Read the model definition and answer for the solid it produces. Units are mm, in the model's axes. A direction names the side the tool comes from. Coordinates: 2 decimals unless noted, no trailing zeros. Loops run counter-clockwise (first coordinate to the right, second up) from the corner with the lowest first, then second, coordinate; pieces in that order, holes last. Notation, with made-up numbers: (66.5, 9.25) -> (105.5, 9.25) arc R18 cw to (105.5, 17.25) -> close; hole circle Ø1 at (46, 35). An arc over 180 degrees is marked (long way). Answer as a JSON object with one key per item and string values. Group by question number.
Q1. The part is cut by section A-A on z = 0. Write down the section's boundary in (x, y).
Q2. The part is cut by section D-D on y = 25. Write down the section's boundary in (x, z), and give its area (3 significant figures).
Q3. Each of these flat-tipped pins is pushed along its axis until it touches: P1, Ø1, axis at x = 7.5, y = -24.5, coming from the +Z side; P2, Ø14, axis at y = -2.5, z = -1, coming from the +X side; P3, Ø8, axis at x = 9, y = -20.5, coming from the +Z side; P4, Ø3, axis at x = 5, y = 0.5, coming from the +Z side. Where does it stop, or does it pass through?
Q4. For faces 1 (the cylindrical face through (5.07, -29.25, 23.53)), 2 (the cylindrical face through (12.958, 27.334, -6.07)), determine the directions among +Z, -Z, +X, -X, +Y, -Y from which every point of the face is accessible in a straight line to the end or side of a thin tool.
Q5. The part is cut by section B-B on y = 0. Write down the section's boundary in (x, z).
Q6. The part is cut by section C-C on z = 35. Write down the section's boundary in (x, y).
Q7. Determine the mould class of faces 3 (the cylindrical face through (5.07, -26.429, -23.033)), 4 (the flat face through (0, 9, -1)), 5 (the cylindrical face through (4.93, 25.861, -33.727)) for opening direction Y: released by +Y, released by -Y, zero draft, split by the parting line, or undercut.
Q8. Straight lines are drawn through the part: line 1 along Y through (x, z) = (13.75, -16.5); line 2 along Y through (x, z) = (13.5, 0); line 3 along Z through (x, y) = (6.25, -31). For each, find the intervals that lie inside material, in ascending order. Write a range as [from, to].
from build123d import *

# Parameters (mm, degrees)
HOLE_WIZARD_6_0_6_1_D = 6.2


with BuildPart() as part:
    # Эскиз1 → Повернуть1 (revolve)
    with BuildSketch(Plane.XY, mode=Mode.PRIVATE) as revolve_1_sk:
        Polygon((0, -2), (8, -2), (8, -23), (16, -23), (16, -28), (10, -28), (10, -42.5), (0, -42.5), align=None)
    revolve(revolve_1_sk.sketch.rotate(Axis((-696.045801993, 0, 0), (1, 0, 0)), 270), axis=Axis((-696.045801993, 0, 0), (1, 0, 0)))

    # Диаметр отверстия Ø6.0 (6)1 (through all)
    with Locations(Plane(origin=(0, 10.815594803, -33.28697807), x_dir=(0, 0, -1), z_dir=(-1, 0, 0))):
        with Locations((0, 0), (-66.57395614, 0), (-33.28697807, -24.184405197), (-12.71449424, 39.131189606), (-53.8594619, 39.131189606)):
            Hole(HOLE_WIZARD_6_0_6_1_D / 2)


solid = part.part
Final values:
{
 "1": {"outline": "(0, -42.5) -> (10, -42.5) -> (10, -28) -> (16, -28) -> (16, -23) -> (8, -23) -> (8, -2) -> (0, -2) -> close; (0, 2) -> (8, 2) -> (8, 23) -> (16, 23) -> (16, 28) -> (10, 28) -> (10, 31.9) -> (0, 31.9) -> close; (0, 38.1) -> (10, 38.1) -> (10, 42.5) -> (0, 42.5) -> close"},
 "2": {"outline": "(0, -34.37) -> (10, -34.37) -> (10, -12.61) -> (16, -12.61) -> (16, 12.61) -> (10, 12.61) -> (10, 34.37) -> (0, 34.37) -> close", "area": "839 mm2"},
 "3": {"P1": "stops at z = 35.07", "P2": "stops at x = 8", "P3": "stops at z = 39.17", "P4": "stops at z = 42.5"},
 "4": {"face 1": "+X, -X", "face 2": "+X"},
 "5": {"outline": "(0, -42.5) -> (10, -42.5) -> (10, -28) -> (16, -28) -> (16, -23) -> (8, -23) -> (8, -2) -> (0, -2) -> close; (0, 2) -> (8, 2) -> (8, 23) -> (16, 23) -> (16, 28) -> (10, 28) -> (10, 42.5) -> (0, 42.5) -> close"},
 "6": {"outline": "(0, -24.11) -> (10, -24.11) -> (10, 8.23) -> (0, 8.23) -> close; (0, 13.4) -> (10, 13.4) -> (10, 24.11) -> (0, 24.11) -> close"},
 "7": {"face 3": "undercut", "face 4": "zero draft", "face 5": "split by the parting line"},
 "8": {"line 1": "y = [-22.62, -16.02], [16.02, 22.62]", "line 2": "y = [-28, -23], [23, 28]", "line 3": "z = [-29.07, -22.12], [-19.02, 19.02], [22.12, 29.07]"}
}
